Geometry: final body of the model. Coordinates: model frame, mm. A direction names the side the tool comes from. Give positions to 0.01 mm unless a question says otherwise; leave off trailing zeros. Order: outer loops, then holes, each group sorted by start corner. A loop starts at its lowest first (then second) coordinate and runs counter-clockwise, first axis right, second up. Notation, with made-up numbers: (18, 39.25) -> (44, 39.25) arc R29 cw to (44, 70.25) -> close; hole circle Ø11 at (61, -33). An arc over 180 degrees is marked (long way). One line per item, written item: value. Start each with the question number.
```python
from build123d import *

# Parameters (mm, degrees)
BOSS_EXTRUDE1_DEPTH = 13
SKETCH2_R           = 1.3
CUT_EXTRUDE1_DEPTH  = 37
FILLET1_R           = 1
FILLET2_R           = 2.6
FILLET3_R           = 4
SKETCH3_R           = 7.86
BOSS_EXTRUDE2_DEPTH = 3
FILLET4_R           = 0.7
BOSS_EXTRUDE3_DEPTH = 7.32
SKETCH6_R           = 0.715
CUT_EXTRUDE2_DEPTH  = 20.35
FILLET5_R           = 0.8


with BuildPart() as part:
    # Sketch1 → Boss-Extrude1 (new body, symmetric)
    with BuildSketch(Plane.XY):
        Polygon((-18, 11.1), (18, 11.1), (18, 0), (15, 0), (15, 7.1), (-15, 7.1), (-15, 0), (-18, 0), align=None)
    extrude(amount=BOSS_EXTRUDE1_DEPTH, both=True)

    # Sketch2 → Cut-Extrude1 (cut, through all)
    with BuildSketch(Plane(origin=(18, 0, 0), x_dir=(0, 0, -1), z_dir=(1, 0, 0))):
        with Locations((-8.5, 2.6)):
            Circle(SKETCH2_R)
        with Locations((8.5, 2.6)):
            Circle(SKETCH2_R)
    extrude(amount=-CUT_EXTRUDE1_DEPTH, mode=Mode.SUBTRACT)

    # Fillet1
    fillet1_edges = [part.edges().sort_by_distance(p)[0] for p in [
        (15, 7.1, 0),
        (-15, 7.1, 0),
    ]]
    fillet(fillet1_edges, radius=FILLET1_R)

    # Fillet2
    fillet2_edges = [part.edges().sort_by_distance(p)[0] for p in [
        (-16.5, 0, -13),
        (16.5, 0, 13),
        (-16.5, 0, 13),
        (16.5, 0, -13),
    ]]
    fillet(fillet2_edges, radius=FILLET2_R)

    # Fillet3
    fillet3_edges = [part.edges().sort_by_distance(p)[0] for p in [
        (-18, 11.1, 0),
        (18, 11.1, 0),
    ]]
    fillet(fillet3_edges, radius=FILLET3_R)

    # Sketch3 → Boss-Extrude2 (add)
    with BuildSketch(Plane(origin=(0, 11.1, 0), x_dir=(1, 0, 0), z_dir=(0, 1, 0))):
        Circle(SKETCH3_R)
    extrude(amount=BOSS_EXTRUDE2_DEPTH)

    # Fillet4
    fillet4_edges = [part.edges().sort_by_distance(p)[0] for p in [
        (-7.86, 11.1, 0),
        (-7.86, 14.1, 0),
    ]]
    fillet(fillet4_edges, radius=FILLET4_R)

    # Sketch5 → Boss-Extrude3 (add)
    with BuildSketch(Plane(origin=(0, 14.1, 0), x_dir=(1, 0, 0), z_dir=(0, 1, 0))):
        with BuildLine():
            Line((1.35, 1.990358008), (1.35, 3.076865288))
            ThreePointArc((1.35, 3.076865288), (0, 3.36), (-1.35, 3.076865288))
            Line((-1.35, 3.076865288), (-1.35, 1.990358008))
            ThreePointArc((-1.35, 1.990358008), (-2.405, 0), (-1.35, -1.990358008))
            Line((-1.35, -1.990358008), (-1.35, -3.076865288))
            ThreePointArc((-1.35, -3.076865288), (0, -3.36), (1.35, -3.076865288))
            Line((1.35, -3.076865288), (1.35, -1.990358008))
            ThreePointArc((1.35, -1.990358008), (2.405, 0), (1.35, 1.990358008))
        make_face()
    extrude(amount=BOSS_EXTRUDE3_DEPTH)

    # Sketch6 → Cut-Extrude2 (cut, through all)
    with BuildSketch(Plane(origin=(1.35, 0, 0), x_dir=(0, 0, -1), z_dir=(1, 0, 0))):
        with Locations((-3.36, 19.47)):
            Circle(SKETCH6_R)
        with Locations((3.36, 19.47)):
            Circle(SKETCH6_R)
    extrude(amount=-CUT_EXTRUDE2_DEPTH, mode=Mode.SUBTRACT)

    # Fillet5
    fillet5_edges = [part.edges().sort_by_distance(p)[0] for p in [
        (0, 21.42, 3.36),
        (0, 21.42, -3.36),
    ]]
    fillet(fillet5_edges, radius=FILLET5_R)


solid = part.part
```
1. Material intervals for L1, parallel to X at y = 1, z = 10.25; L2, parallel to Z at x = 16, y = 1.5; L3, parallel to Y at x = -9.5, z = -10, sorted ascending. Write a range as [from, to].
2. Cut plane A-A, the plane y = 4.75. Return loops of the section in (x, z).
3. Cut plane C-C, the plane z = -11. Return loops of the section in (x, y), then the cut area to 3 significant figures.
4. Access query for faces 1 (the flat face through (-1.35, 17.7, 2.5)), 2 (the cylindrical face through (-1.704, 12.589, 7.673)), 3 (the flat face through (-15, 3, 0)). Directions: +Z, -Z, +X, -X, +Y, -Y. A direction counts if a zero-diameter tool reaches every point of the face in a straight line with its end or side. Return the directions, or none.
5. Draft query along Y for faces 4 (the cylindrical face through (-2.405, 17.709, -0.033)), 5 (the cylindrical face through (0.019, 19.486, -2.645)), 6 (the cylindrical face through (16.479, 0.741, 12.218)). Return one class per face: pulls with the +Y half, pulls with the -Y half, needs draft (parallel to the pull), parting line crosses it, or undercut.
6. Cut plane B-B, the plane x = 0. Return loops of the section in (y, z) (3 decimals).
7. Pin query (flat end, axial travel): P1, Ø1.2, axis at y = 18.5, z = 2.5, coming from the -X side; P2, Ø0.5, axis at y = 17.5, z = 2.5, coming from the +X side; P3, Ø13, axis at x = 2.5, z = -2.5, coming from the -Y side. Return the tip coordinate at first contact, or that it passes through.
8. Cut plane D-D, the plane y = 19.47. Return loops of the section in (x, z) (3 decimals), then the cut area to 3 significant figures.
Answers follow:
1. L1: x = [-18, -15], [15, 18]
1. L2: z = [-12.76, -9.19], [-7.81, 7.81], [9.19, 12.76]
1. L3: y = [7.1, 11.1]
2. outline: (-18, -13) -> (-15, -13) -> (-15, 13) -> (-18, 13) -> close; (15, -13) -> (18, -13) -> (18, 13) -> (15, 13) -> close
3. outline: (-18, 0.07) -> (-15, 0.07) -> (-15, 6.1) arc R1 cw to (-14, 7.1) -> (14, 7.1) arc R1 cw to (15, 6.1) -> (15, 0.07) -> (18, 0.07) -> (18, 7.1) arc R4 ccw to (14, 11.1) -> (-14, 11.1) arc R4 ccw to (-18, 7.1) -> close
3. area: 180 mm²
4. face 1: +Z, -X, +Y
4. face 2: +Y
4. face 3: +Z, -Z, -Y
5. face 4: needs draft
5. face 5: undercut
5. face 6: pulls with the -Y half
6. outline: (7.1, -13) -> (11.1, -13) -> (11.1, -8.56) arc R0.7 cw to (11.8, -7.86) -> (13.4, -7.86) arc R0.7 ccw to (14.1, -7.16) -> (14.1, -3.36) -> (18.755, -3.36) arc R0.715 cw to (20.185, -3.36) -> (20.62, -3.36) arc R0.8 ccw to (21.42, -2.56) -> (21.42, 2.56) arc R0.8 ccw to (20.62, 3.36) -> (20.185, 3.36) arc R0.715 cw to (18.755, 3.36) -> (14.1, 3.36) -> (14.1, 7.16) arc R0.7 ccw to (13.4, 7.86) -> (11.8, 7.86) arc R0.7 cw to (11.1, 8.56) -> (11.1, 13) -> (7.1, 13) -> close
7. P1: stops at x = -1.47
7. P2: stops at x = 1.35
7. P3: stops at y = 7.1
8. outline: (-1.35, -2.645) -> (1.35, -2.645) -> (1.35, -1.99) arc R2.405 ccw to (1.35, 1.99) -> (1.35, 2.645) -> (-1.35, 2.645) -> (-1.35, 1.99) arc R2.405 ccw to (-1.35, -1.99) -> close
8. area: 20.2 mm²
